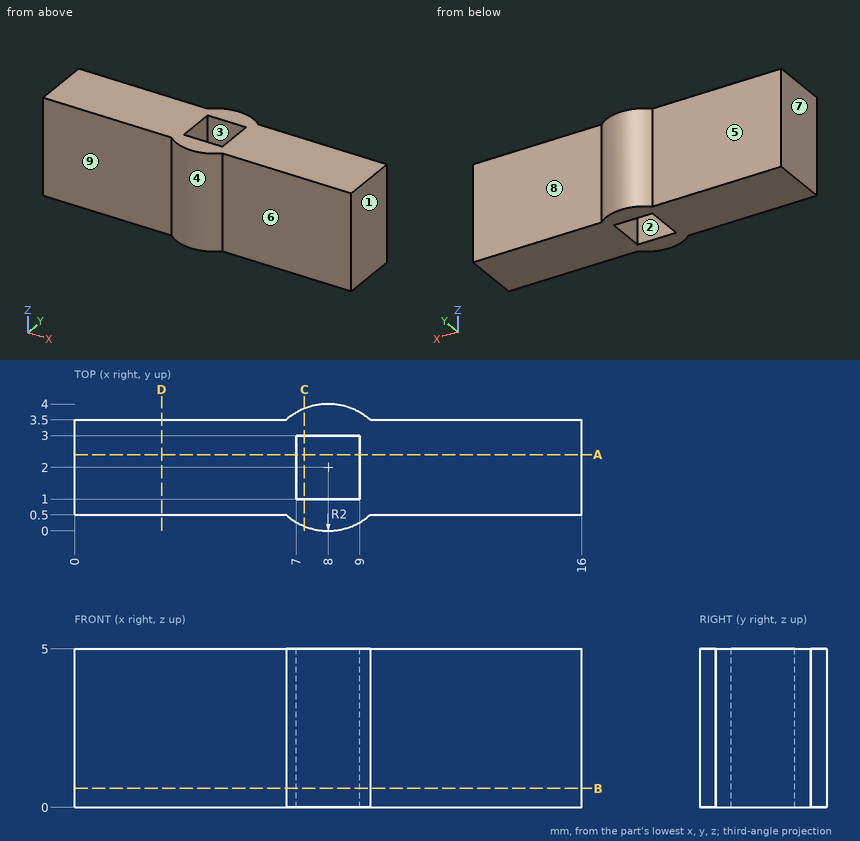
The drawing under review shows one solid part. Ordinate dimensions are in mm from its lowest x, y, z. A direction names the side the tool comes from. Coordinates: 2 decimals unless noted, no trailing zeros. Order: outer loops, then holes, each group sorted by start corner. A loop starts at its lowest first (then second) coordinate and runs counter-clockwise, first axis right, second up. Notation, with made-up numbers: (80, 30.25) - (101, 30.25) arc R13 ccw to (101, 39.25) - close; hole circle Ø9 at (43.5, 60.5). An arc over 180 degrees is marked (long way). Put each result on its own line as item: value.
1) Insertion check: P1, Ø1.5, axis at x = 6, z = 3.5, coming from the +Y side; P2, Ø0.6, axis at x = 8.5, z = 3, coming from the +Y side; P3, Ø2.5, axis at x = 3, z = 2, coming from the +Y side. Each pin has a flat end and moves straight along its axis. Give the tip position at first contact, or say it passes through.
Response values:
P1: stops at y = 3.56
P2: stops at y = 3.99
P3: stops at y = 3.5
2) Take a section at A-A, the plane y = 2.4. Give the boundary of the cut face in (x, z).
Response values:
outline: (0, 0) - (7, 0) - (7, 5) - (0, 5) - close; (9, 0) - (16, 0) - (16, 5) - (9, 5) - close
3) Tool access review of the marked faces 5, 6, 7, 8 and 9: name each direction out of +Z, -Z, +X, -X, +Y, -Y from which nothing blocks a thin tool from reaching the whole face with its end or side.
Response values:
face 5: +Z, -Z, -X, +Y
face 6: +Z, -Z, +X, -Y
face 7: +Z, -Z, -X, +Y, -Y
face 8: +Z, -Z, +X, +Y
face 9: +Z, -Z, -X, -Y
4) Wall thickness on L1, parallel to X at y = 1.8, z = 1.1; L2, parallel to Y at x = 3.5, z = 4.1; L3, parallel to Y at x = 7.25, z = 0.8: over which ranges is each line inside the solid? List them lowest first. Write a range as from..to.
Response values:
L1: x = 0..7, 9..16
L2: y = 0.5..3.5
L3: y = 0.15..1, 3..3.85
5) Take a section at C-C, the plane x = 7.25. Give the boundary of the cut face in (y, z).
Response values:
outline: (0.15, 0) - (1, 0) - (1, 5) - (0.15, 5) - close; (3, 0) - (3.85, 0) - (3.85, 5) - (3, 5) - close
6) The part is to be moulded in two halves that separate along Y. For the marked faces 1, 2, 3 and 4, say which applies: released by +Y, released by -Y, zero draft, split by the parting line, or undercut.
Response values:
face 1: zero draft
face 2: undercut
face 3: undercut
face 4: released by -Y
7) Take a section at D-D, the plane x = 2.75. Give the boundary of the cut face in (y, z).
Response values:
outline: (0.5, 0) - (3.5, 0) - (3.5, 5) - (0.5, 5) - close
8) Take a section at B-B, the plane z = 0.6. Give the boundary of the cut face in (x, y), and give its area (3 significant figures).
Response values:
outline: (0, 0.5) - (6.68, 0.5) arc R2 ccw to (9.32, 0.5) - (16, 0.5) - (16, 3.5) - (9.32, 3.5) arc R2 ccw to (6.68, 3.5) - (0, 3.5) - close; hole (7, 1) - (9, 1) - (9, 3) - (7, 3) - close
area: 45.8 mm²
